```python
from build123d import *

# Parameters (mm, degrees)
SKETCH1_W           = 130
SKETCH1_H           = 430
BOSS_EXTRUDE1_DEPTH = 3
SKETCH2_W           = 42
SKETCH2_H           = 40
CUT_EXTRUDE1_DEPTH  = 10
SKETCH3_R           = 1.5
SKETCH3_R_2         = 2.1
CUT_EXTRUDE2_DEPTH  = 10
SKETCH4_R           = 7
CUT_EXTRUDE3_DEPTH  = 10
SKETCH5_R           = 4
SKETCH5_R_2         = 1.25
CUT_EXTRUDE4_DEPTH  = 10


with BuildPart() as part:
    # Sketch1 → Boss-Extrude1 (new body)
    with BuildSketch(Plane(origin=(0, 0, 0), x_dir=(1, 0, 0), z_dir=(0, 1, 0))):
        Rectangle(SKETCH1_W, SKETCH1_H)
    extrude(amount=BOSS_EXTRUDE1_DEPTH)

    # Sketch2 → Cut-Extrude1 (cut)
    with BuildSketch(Plane(origin=(0, 3, 0), x_dir=(1, 0, 0), z_dir=(0, 1, 0))):
        with Locations((0, -195)):
            Rectangle(SKETCH2_W, SKETCH2_H)
    extrude(amount=-CUT_EXTRUDE1_DEPTH, mode=Mode.SUBTRACT)

    # Sketch3 → Cut-Extrude2 (cut)
    with BuildSketch(Plane.XZ):
        with Locations(Location((-53.05, -3.75, 0), (0, 0, 270))):
            Circle(SKETCH3_R)
        with Locations(Location((-24.95, -3.75, 0), (0, 0, 270))):
            Circle(SKETCH3_R)
        with Locations(Location((-53.05, -106.75, 0), (0, 0, 270))):
            Circle(SKETCH3_R)
        with Locations(Location((-24.95, -106.75, 0), (0, 0, 270))):
            Circle(SKETCH3_R)
        with Locations(Location((24.95, -106.75, 0), (0, 0, 90))):
            Circle(SKETCH3_R)
        with Locations(Location((34, 195, 0), (0, 0, 270))):
            Circle(SKETCH3_R_2)
        with Locations(Location((53.05, -106.75, 0), (0, 0, 90))):
            Circle(SKETCH3_R)
        with Locations(Location((24.95, -3.75, 0), (0, 0, 90))):
            Circle(SKETCH3_R)
        with Locations(Location((-34, 195, 0), (0, 0, 270))):
            Circle(SKETCH3_R_2)
        with Locations(Location((53.05, -3.75, 0), (0, 0, 90))):
            Circle(SKETCH3_R)
        with Locations(Location((-41.5, 175, 0), (0, 0, 270))):
            Circle(SKETCH3_R_2)
        with Locations(Location((41.5, 175, 0), (0, 0, 270))):
            Circle(SKETCH3_R_2)
        with Locations(Location((41.5, -175, 0), (0, 0, 270))):
            Circle(SKETCH3_R_2)
        with Locations(Location((-41.5, -175, 0), (0, 0, 270))):
            Circle(SKETCH3_R_2)
    extrude(amount=-CUT_EXTRUDE2_DEPTH, mode=Mode.SUBTRACT)

    # Sketch4 → Cut-Extrude3 (cut)
    with BuildSketch(Plane.XZ):
        with Locations(Location((-17.5, 115, 0), (0, 0, 270))):
            Circle(SKETCH4_R)
        with Locations(Location((17.5, 115, 0), (0, 0, 270))):
            Circle(SKETCH4_R)
    extrude(amount=-CUT_EXTRUDE3_DEPTH, mode=Mode.SUBTRACT)

    # Sketch5 → Cut-Extrude4 (cut)
    with BuildSketch(Plane.XZ):
        with Locations(Location((-15, -75, 0), (0, 0, 270))):
            Circle(SKETCH5_R)
        with Locations(Location((-14, -86, 0), (0, 0, 270))):
            Circle(SKETCH5_R_2)
        with Locations(Location((-5, -86, 0), (0, 0, 270))):
            Circle(SKETCH5_R_2)
        with Locations(Location((-15, 75, 0), (0, 0, 90))):
            Circle(SKETCH5_R)
        with Locations(Location((-14, 86, 0), (0, 0, 90))):
            Circle(SKETCH5_R_2)
        with Locations(Location((-5, 86, 0), (0, 0, 90))):
            Circle(SKETCH5_R_2)
    extrude(amount=-CUT_EXTRUDE4_DEPTH, mode=Mode.SUBTRACT)


solid = part.part
```
Check sheet for the modelled part. Datum: model origin and axes. Units: mm. Coordinates: 2 decimals unless noted, no trailing zeros. Use one line per item in the form item = value.
Item 1: Sectioned sample at A-A, the plane y = 1.65. State how many separate pieces and enclosed holes the cut face has, and give its area (3 significant figures).
Answer below:
separate_pieces = 1
enclosed_holes = 22
area = 53,700 mm^2
Item 2: Release check for a two-part mould opening along Z. For faces 1 (the face through (-1, 0, -3)), 2 (the face through (-17.192, 1.479, 121.993)) record: pulls with the +Z half, pulls with the -Z half, needs draft (parallel to the pull), parting line crosses it, or undercut.
Answer below:
face_1 = needs draft
face_2 = undercut
Item 3: Material ranges on L1, parallel to Z at x = 53.05, y = 1.7; L2, parallel to X at y = 0.65, z = 195; L3, parallel to X at y = 1.6, z = -86, recorded low to high. Write a range as from..to.
Answer below:
L1 = -215..-108.25, -105.25..-5.25, -2.25..215
L2 = -65..-36.1, -31.9..-21, 21..31.9, 36.1..65
L3 = -65..-15.25, -12.75..-6.25, -3.75..65
Item 4: Gauge pin test, flat end, axial feed: pin 1 Ø1.5 at (x, y) = (-9.5, 1.5) entering from +Z. Record the tip position at first contact, or that the pin passes through.
Answer below:
pin_1 = 175
